Check sheet for the drawn part. Datum: minimum x, y, z corner. Units: mm. A direction names the side the tool comes from. Give positions to 0.01 mm unless a question says otherwise; leave off trailing zeros. Order: outer loops, then holes, each group sorted by start corner. A loop starts at its lowest first (then second) coordinate and runs counter-clockwise, first axis right, second up. Notation, with made-up numbers: (-27, -28.5) -> (9, -28.5) arc R7 ccw to (9, -24.5) -> close; hole circle Ø9 at (-15.5, -26.75). An arc over 180 degrees is marked (long way). Return JSON: item names as keys, results as strings. Group by question number.
(1) Tool access check on the marked faces 4 and 5. Record the directions out of +Z, -Z, +X, -X, +Y, -Y that give a thin tool (end or side, any length) a straight path to the whole face; none if there is none.
(2) Thickness scan on line 1 along X through (y, z) = (17.5, 2.65); line 2 along X through (y, z) = (14, 2.95). Record the ranges inside material, lowest first.
(3) Cross-section at C-C on y = 25. Enter the section's corners in (x, z) (1 decimal), then the cut area to 3 significant figures.
(4) Release check for a two-part mould opening along X. For the marked faces 1, 2 and 3 record: pulls with the +X half, pulls with the -X half, needs draft (parallel to the pull), parting line crosses it, or undercut.
(5) Cross-section at A-A on x = 19.5. Enter the section's corners in (y, z) (1 decimal).
(6) Cross-section at B-B on z = 0.4. Enter the section's corners in (x, y) (1 decimal).
(7) Cross-section at D-D on x = 5.5. Enter the section's corners in (y, z) (1 decimal).
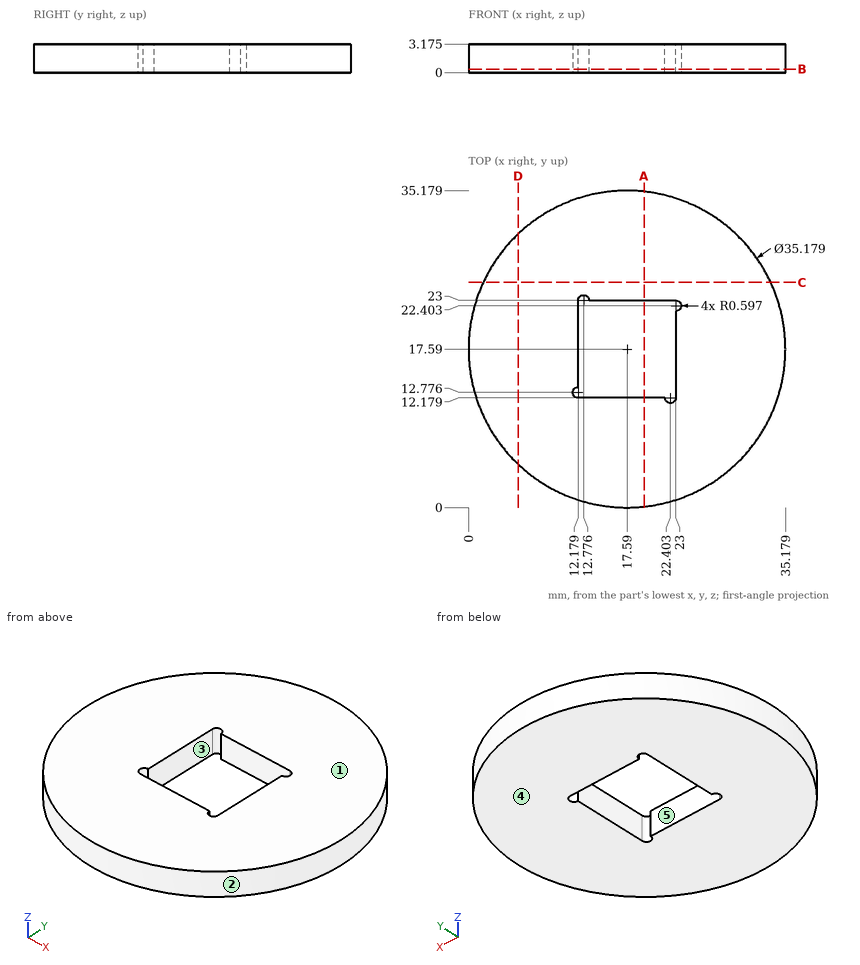
Verdict:
{
 "1": {"face 4": "-Z, +X, -X, +Y, -Y", "face 5": "+Z, -Z"},
 "2": {"line 1": "0 to 12.18, 23 to 35.18", "line 2": "0.37 to 12.18, 23 to 34.81"},
 "3": {"outline": "(1.6, 0) -> (33.5, 0) -> (33.5, 3.2) -> (1.6, 3.2) -> close", "area": "101 mm²"},
 "4": {"face 1": "needs draft", "face 2": "parting line crosses it", "face 3": "undercut"},
 "5": {"outline": "(0.1, 0) -> (12.2, 0) -> (12.2, 3.2) -> (0.1, 3.2) -> close; (23, 0) -> (35.1, 0) -> (35.1, 3.2) -> (23, 3.2) -> close"},
 "6": {"outline": "circle Ø35.2 at (17.6, 17.6); hole (12.2, 12.2) -> (21.8, 12.2) arc R0.6 ccw to (23, 12.2) -> (23, 21.8) arc R0.6 ccw to (23, 23) -> (13.4, 23) arc R0.6 ccw to (12.2, 23) -> (12.2, 13.4) arc R0.6 ccw to start"},
 "7": {"outline": "(4.8, 0) -> (30.4, 0) -> (30.4, 3.2) -> (4.8, 3.2) -> close"}
}
